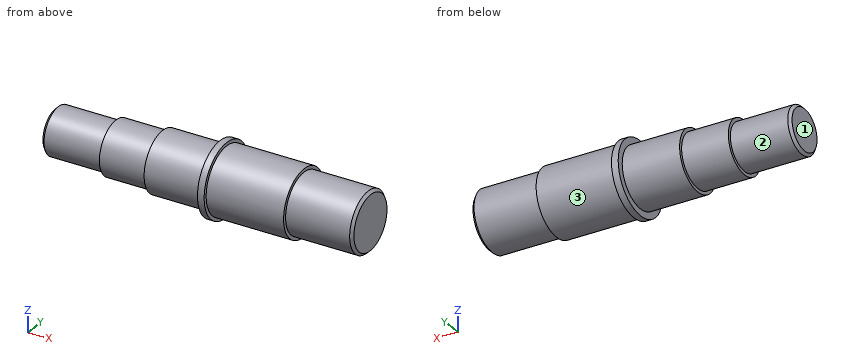
Autodesk Inventor part; units mm, degrees
ref_plane "Start Plane" through (0, 0, 0) normal (1, 0, 0) x (0, 1, 0)
ref_plane "XZ Plane" through (0, 0, 0) normal (0, 1, 0) x (-1, 0, 0)
ref_plane "XY Plane" through (0, 0, 0) normal (0, 0, 1) x (1, 0, 0)
sketch "Main Sketch" plane through (0, 0, 0) normal (0, 0, 1) x (1, 0, 0)
  line L0 (0, 0) -> (236, 0)
  line L1 (0, 0) -> (0, 17.5)
  line L2 (0, 17.5) -> (45, 17.5)
  line L3 (45, 17.5) -> (45, 20)
  line L4 (45, 20) -> (80, 20)
  line L5 (80, 20) -> (80, 22.5)
  line L6 (80, 22.5) -> (123, 22.5)
  line L7 (123, 22.5) -> (123, 27.5)
  line L8 (128, 27.5) -> (128, 25)
  line L9 (123, 27.5) -> (128, 27.5)
  line L10 (186, 25) -> (186, 22.5)
  line L11 (128, 25) -> (186, 25)
  line L12 (236, 22.5) -> (236, 0)
  line L13 (186, 22.5) -> (236, 22.5)
  dimension "d3" = 35
  dimension "d4" = 40
  dimension "d5" = 45
  dimension "d6" = 55
  dimension "d7" = 50
  dimension "d8" = 45
revolve "Revolution1" add sketch "Main Sketch" angle 360 about axis through (0, 0, 0) along (1, 0, 0)
chamfer "Chamfer1" distance 2 angle 45 1 edges at (0, -17.5, 0) measured on face at (30, 17.2734, -2.8072)
chamfer "Chamfer2" distance 2 angle 45 1 edges at (236, -22.5, 0) measured on face at (219.3333, 22.2086, -3.6093)
equation "\"Length\" = 236"
properties part number "Shaft" material "Steel"
For this review, take the finished solid that the model builds, in its own axes (mm). Face numbers are marked on the shaded views. A direction names the side the tool comes from. Give positions to 0.01 mm unless a question says otherwise; leave off trailing zeros. Write each loop counter-clockwise with the first axis right and the second up, starting at its lowest first coordinate (ties: lowest second). Pieces come first, ordered by that corner, then holes. Notation, with made-up numbers: M -4.75,-33.5 L 37.25,-33.5 A14 ccw 37.25,-22.5 Z; hole C 80,-22 d9. An arc over 180 degrees is marked long. Answer as a JSON object with one key per item and string values. Group by question number.
Item 1: Consider section A-A on y = 0. Write out the cut boundary in (x, z).
Item 2: Tool access review of the marked faces 1, 2 and 3: name each direction out of +Z, -Z, +X, -X, +Y, -Y from which nothing blocks a thin tool from reaching the whole face with its end or side.
Item 3: Consider section C-C on x = 210. Write out the cut boundary in (y, z).
Item 4: Consider section D-D on x = 36.5. Write out the cut boundary in (y, z), plus the area to 3 significant figures.
Item 5: For pin 1 Ø1.5 at (x, y) = (188.5, -6.5) entering from -Z; pin 2 Ø6 at (x, y) = (114, 13.5) entering from +Z; pin 3 Ø2 at (x, z) = (189, -10.5) entering from +Y, all flat-tipped, find the tip position at first contact; note any pin that passes through.
Item 6: For probe 1 along Y at (x, z) = (139, 1); probe 2 along Y at (x, z) = (112.5, -1); probe 3 along X at (y, z) = (17.5, -5), list the stretches that pass through material, from the lowest coordinate up. Write a range as [from, to].
Check result:
{
 "1": {"outline": "M 0,-15.5 L 2,-17.5 L 45,-17.5 L 45,-20 L 80,-20 L 80,-22.5 L 123,-22.5 L 123,-27.5 L 128,-27.5 L 128,-25 L 186,-25 L 186,-22.5 L 234,-22.5 L 236,-20.5 L 236,20.5 L 234,22.5 L 186,22.5 L 186,25 L 128,25 L 128,27.5 L 123,27.5 L 123,22.5 L 80,22.5 L 80,20 L 45,20 L 45,17.5 L 2,17.5 L 0,15.5 Z"},
 "2": {"face 1": "+Z, -Z, -X, +Y, -Y", "face 2": "-X", "face 3": "+X"},
 "3": {"outline": "C 0,0 d45"},
 "4": {"outline": "C 0,0 d35", "area": "962 mm^2"},
 "5": {"pin 1": "stops at z = -21.75", "pin 2": "stops at z = 19.9", "pin 3": "stops at y = 20.4"},
 "6": {"probe 1": "y = [-24.98, 24.98]", "probe 2": "y = [-22.48, 22.48]", "probe 3": "x = [45, 236]"}
}
